Check sheet for the drawn part. Datum: minimum x, y, z corner. Units: mm. A direction names the side the tool comes from. Give positions to 0.01 mm unless a question says otherwise; leave off trailing zeros. Order: outer loops, then holes, each group sorted by start corner. A loop starts at its lowest first (then second) coordinate and runs counter-clockwise, first axis right, second up. Notation, with made-up numbers: (76.25, -5) - (121.25, -5) arc R19 cw to (121.25, 19) - close; hole circle Ø4 at (73.25, 21). An arc over 180 degrees is marked (long way). Answer as a JSON object with one key per item and string values. Group by question number.
(1) Mould release check, pull along Y, two halves, no side actions. Record for the marked faces 3, 4 and 5: +Y half, -Y half, draft (parallel to the pull), parting line (faces both ways), or undercut.
(2) Depth check by flat-ended pin: pin 1 Ø1.5 at (x, z) = (3.5, 6.5) entering from -Y; pin 2 Ø2 at (x, z) = (2, 2.5) entering from +Y; pin 3 Ø3 at (x, z) = (3, 3) entering from -Y. Enter the tip coordinate at first touch or a pass-through.
(3) Thickness scan on line 1 (Z direction, x = 2.5, y = 11.75); line 2 (Y direction, x = 7.75, z = 2.25); line 3 (Y direction, x = 7.62, z = 4.5) (3 decimals). Record the ranges inside material, lowest first.
(4) Section check A-A (y = 7.62). Record the boundary of the cut face in (x, z) (3 decimals).
(5) Section check C-C (x = 12.75). Record the boundary of the cut face in (y, z), then the cut area to 3 significant figures.
(6) Access from +Z, -Z, +X, -X, +Y, -Y to the whole of each face (thin tool, end or side, straight path). Record for the marked faces 1 and 2.
(7) Section check D-D (z = 5.75). Record the boundary of the cut face in (x, y) (3 decimals), then the cut area to 3 significant figures.
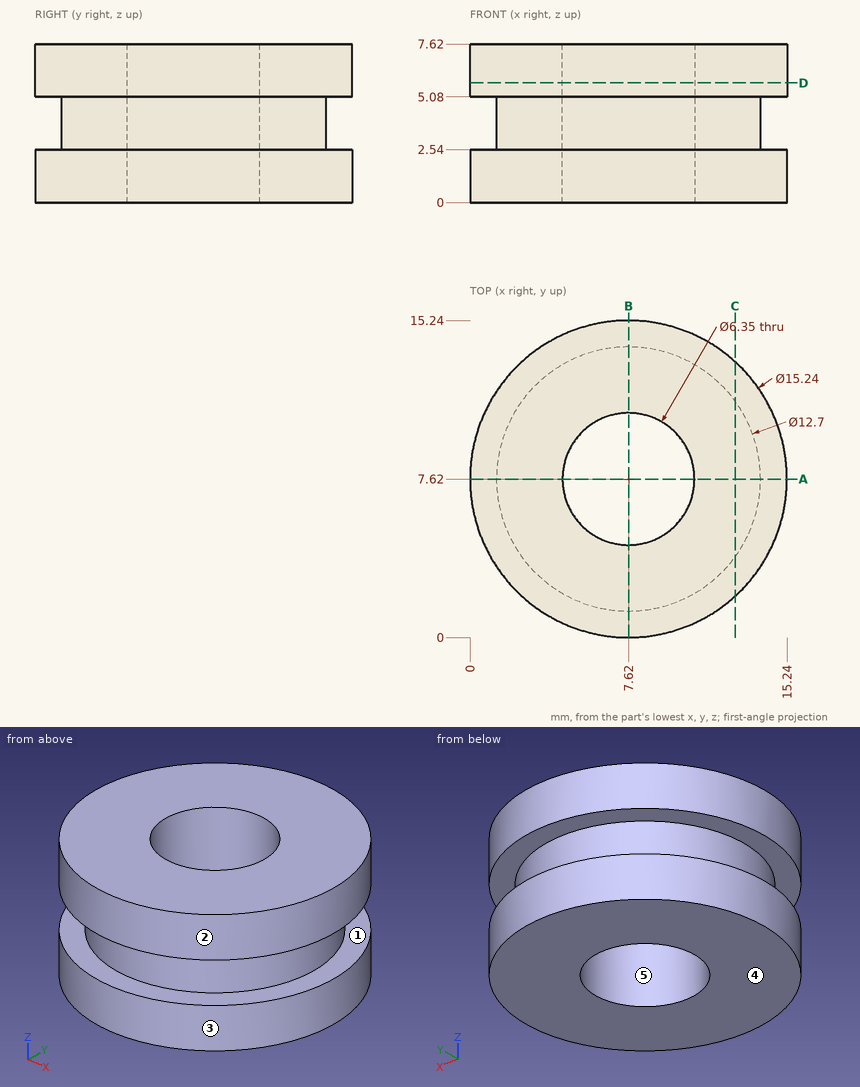
Solutions:
{
 "1": {"face 3": "parting line", "face 4": "draft", "face 5": "undercut"},
 "2": {"pin 1": "stops at y = 0.79", "pin 2": "stops at y = 13.68", "pin 3": "stops at y = 0.7"},
 "3": {"line 1": "z = 0 to 2.54, 5.08 to 7.62", "line 2": "y = 0 to 4.45, 10.79 to 15.24", "line 3": "y = 1.27 to 4.445, 10.795 to 13.97"},
 "4": {"outline": "(0, 0) - (4.445, 0) - (4.445, 7.62) - (0, 7.62) - (0, 5.08) - (1.27, 5.08) - (1.27, 2.54) - (0, 2.54) - close; (10.795, 0) - (15.24, 0) - (15.24, 2.54) - (13.97, 2.54) - (13.97, 5.08) - (15.24, 5.08) - (15.24, 7.62) - (10.795, 7.62) - close"},
 "5": {"outline": "(1.99, 0) - (13.25, 0) - (13.25, 2.54) - (11.36, 2.54) - (11.36, 5.08) - (13.25, 5.08) - (13.25, 7.62) - (1.99, 7.62) - (1.99, 5.08) - (3.88, 5.08) - (3.88, 2.54) - (1.99, 2.54) - close", "area": "76.3 mm2"},
 "6": {"face 1": "none", "face 2": "+Z, -Z"},
 "7": {"outline": "circle Ø15.24 at (7.62, 7.62); hole circle Ø6.35 at (7.62, 7.62)", "area": "151 mm2"}
}
